```python
from build123d import *

# Parameters (mm, degrees)
SKETCH7_W           = 100
SKETCH7_H           = 14.5
BOSS_EXTRUDE1_DEPTH = 16.5
SKETCH8_R           = 4.75
CUT_EXTRUDE2_DEPTH  = 16
CUT_EXTRUDE3_START  = -2
SKETCH9_W           = 27
SKETCH9_H           = 27
CUT_EXTRUDE3_DEPTH  = 2
CUT_EXTRUDE4_DEPTH  = 2
FILLET1_R           = 3
FILLET2_R           = 3
FILLET3_R           = 0.3
FILLET4_R           = 3


with BuildPart() as part:
    # Sketch7 → Boss-Extrude1 (new body)
    with BuildSketch(Plane(origin=(0, 0, 0), x_dir=(0, 1, 0), z_dir=(0, 0, 1))):
        Rectangle(SKETCH7_W, SKETCH7_H)
    extrude(amount=BOSS_EXTRUDE1_DEPTH)

    # Sketch8 → Cut-Extrude2 (cut)
    with BuildSketch(Plane(origin=(0, 0, 16.5), x_dir=(0, -1, 0), z_dir=(0, 0, 1))):
        with Locations(Location((0, 0, 0), (0, 0, 90))):
            Circle(SKETCH8_R)
    extrude(amount=-CUT_EXTRUDE2_DEPTH, mode=Mode.SUBTRACT)

    # Sketch9 → Cut-Extrude3 (cut)
    with BuildSketch(Plane.XY.offset(16.5).offset(CUT_EXTRUDE3_START)):
        with Locations((0, -35)):
            Rectangle(SKETCH9_W, SKETCH9_H)
    cut_extrude3 = extrude(amount=-CUT_EXTRUDE3_DEPTH, mode=Mode.SUBTRACT)

    # Sketch10 → Cut-Extrude4 (cut)
    with BuildSketch(Plane.XY.offset(16.5)):
        with BuildLine():
            Line((0, -28), (-7.25, -28))
            Line((-7.25, -28), (-7.25, -42))
            Line((-7.25, -42), (0, -42))
            ThreePointArc((0, -42), (7, -35), (0, -28))
        make_face()
    cut_extrude4 = extrude(amount=-CUT_EXTRUDE4_DEPTH, mode=Mode.SUBTRACT)

    # Mirror1: Cut-Extrude3 across plane
    add(cut_extrude3.mirror(Plane.ZX), mode=Mode.SUBTRACT)

    # Mirror2: Cut-Extrude4 across plane
    add(cut_extrude4.mirror(Plane.ZX), mode=Mode.SUBTRACT)

    # Fillet1
    fillet1_edges = [part.edges().sort_by_distance(p)[0] for p in [
        (-7.25, 0, 0),
    ]]
    fillet(fillet1_edges, radius=FILLET1_R)

    # Fillet2
    fillet2_edges = [part.edges().sort_by_distance(p)[0] for p in [
        (7.25, 0, 0),
    ]]
    fillet(fillet2_edges, radius=FILLET2_R)

    # Fillet3
    fillet3_edges = [part.edges().sort_by_distance(p)[0] for p in [
        (-4.75, 0, 16.5),
    ]]
    fillet(fillet3_edges, radius=FILLET3_R)

    # Fillet4
    # the kernel refuses this fillet: 3 mm, written as the material it takes off along each edge
    with BuildSketch(Plane(origin=(-4.25, -50, 3), x_dir=(0, 0, -1), z_dir=(1, 0, 0))) as fillet4_piece_1:
        with BuildLine():
            CenterArc((3 - FILLET4_R, FILLET4_R), FILLET4_R, 270, 90)
            Line((3, FILLET4_R), (3, 0))
            Line((3, 0), (3 - FILLET4_R, 0))
        make_face()
    revolve(axis=Axis((-4.25, -50, 3), (0, 1, 0)), revolution_arc=90, mode=Mode.SUBTRACT)
    with BuildSketch(Plane(origin=(-7.25, -50, 3), x_dir=(0, 1, 0), z_dir=(0, 0, 1))) as fillet4_piece_2:
        with BuildLine():
            CenterArc((FILLET4_R, -FILLET4_R), FILLET4_R, 90, 90)
            Line((0, -FILLET4_R), (0, 0))
            Line((0, 0), (FILLET4_R, 0))
        make_face()
    extrude(amount=21, mode=Mode.SUBTRACT)
    with BuildSketch(Plane(origin=(-14.75, -50, 16.5), x_dir=(0, 1, 0), z_dir=(1, 0, 0)), Plane(origin=(14.75, 50, 16.5), x_dir=(0, -1, 0), z_dir=(-1, 0, 0))) as fillet4_piece_3:
        with BuildLine():
            CenterArc((FILLET4_R, -FILLET4_R), FILLET4_R, 90, 90)
            Line((0, -FILLET4_R), (0, 0))
            Line((0, 0), (FILLET4_R, 0))
        make_face()
    extrude(amount=29.5, mode=Mode.SUBTRACT)
    with BuildSketch(Plane(origin=(7.25, -50, 3), x_dir=(0, 1, 0), z_dir=(0, 0, 1)), Plane(origin=(-7.25, 50, 3), x_dir=(0, -1, 0), z_dir=(0, 0, 1)), Plane(origin=(7.25, 50, 3), x_dir=(-1, 0, 0), z_dir=(0, 0, 1))) as fillet4_piece_4:
        with BuildLine():
            CenterArc((FILLET4_R, FILLET4_R), FILLET4_R, 180, 90)
            Line((0, FILLET4_R), (0, 0))
            Line((0, 0), (FILLET4_R, 0))
        make_face()
    extrude(amount=21, mode=Mode.SUBTRACT)
    with BuildSketch(Plane(origin=(4.25, -50, 3), x_dir=(0, 0, -1), z_dir=(-1, 0, 0))) as fillet4_piece_5:
        with BuildLine():
            CenterArc((3 - FILLET4_R, -FILLET4_R), FILLET4_R, 0, 90)
            Line((3, -FILLET4_R), (3, 0))
            Line((3, 0), (3 - FILLET4_R, 0))
        make_face()
    revolve(axis=Axis((4.25, -50, 3), (0, -1, 0)), revolution_arc=90, mode=Mode.SUBTRACT)
    with BuildSketch(Plane(origin=(-4.25, -50, 0), x_dir=(0, 0, 1), z_dir=(1, 0, 0)), Plane(origin=(4.25, 50, 0), x_dir=(0, 0, 1), z_dir=(-1, 0, 0))) as fillet4_piece_6:
        with BuildLine():
            CenterArc((FILLET4_R, -FILLET4_R), FILLET4_R, 90, 90)
            Line((0, -FILLET4_R), (0, 0))
            Line((0, 0), (FILLET4_R, 0))
        make_face()
    extrude(amount=8.5, mode=Mode.SUBTRACT)
    with BuildSketch(Plane(origin=(-4.25, 50, 3), x_dir=(0, 0, -1), z_dir=(1, 0, 0))) as fillet4_piece_7:
        with BuildLine():
            CenterArc((3 - FILLET4_R, -FILLET4_R), FILLET4_R, 0, 90)
            Line((3, -FILLET4_R), (3, 0))
            Line((3, 0), (3 - FILLET4_R, 0))
        make_face()
    revolve(axis=Axis((-4.25, 50, 3), (0, 1, 0)), revolution_arc=90, mode=Mode.SUBTRACT)
    with BuildSketch(Plane(origin=(4.25, 50, 3), x_dir=(0, 0, -1), z_dir=(-1, 0, 0))) as fillet4_piece_8:
        with BuildLine():
            CenterArc((3 - FILLET4_R, FILLET4_R), FILLET4_R, 270, 90)
            Line((3, FILLET4_R), (3, 0))
            Line((3, 0), (3 - FILLET4_R, 0))
        make_face()
    revolve(axis=Axis((4.25, 50, 3), (0, -1, 0)), revolution_arc=90, mode=Mode.SUBTRACT)


solid = part.part
```
Geometry: final body of the model. Coordinates: model frame, mm. A direction names the side the tool comes from. Coordinates: 2 decimals unless noted, no trailing zeros. Order: outer loops, then holes, each group sorted by start corner. A loop starts at its lowest first (then second) coordinate and runs counter-clockwise, first axis right, second up. Notation, with made-up numbers: (73, 32) -> (113, 32) arc R25 cw to (113, 53) -> close; hole circle Ø7 at (23.25, 44.25). An arc over 180 degrees is marked (long way). Answer in a Markdown table with one row per item.
Item 1: Section C-C on y = 12. Output: boundary loops of the cut face in (x, z), plus the area to 3 significant figures.
Return value:
| item | result |
|---|---|
| outline | (-7.25, 3) arc R3 ccw to (-4.25, 0) -> (4.25, 0) arc R3 ccw to (7.25, 3) -> (7.25, 16.5) -> (-7.25, 16.5) -> close |
| area | 235 mm² |
Item 2: Section B-B on y = 35. Output: boundary loops of the cut face in (x, z), plus the area to 3 significant figures.
Return value:
| item | result |
|---|---|
| outline | (-7.25, 3) arc R3 ccw to (-4.25, 0) -> (4.25, 0) arc R3 ccw to (7.25, 3) -> (7.25, 12.5) -> (-7.25, 12.5) -> close; (7, 14.5) -> (7.25, 14.5) -> (7.25, 16.5) -> (7, 16.5) -> close |
| area | 178 mm² |
Item 3: Contact query for flat-ended pins moving along their axis: P1, Ø2, axis at x = -4, z = 16, coming from the +Y side; P2, Ø1, axis at x = -2.5, z = 15.5, coming from the -Y side; P3, Ø2, axis at x = -2.5, z = 15.5, coming from the -Y side. Output: stop coordinate, or through.
Return value:
| item | result |
|---|---|
| P1 | stops at y = 49.6 |
| P2 | stops at y = -49.6 |
| P3 | stops at y = -49.83 |
Item 4: Draft query along Z for faces 4 (the flat face through (0, 50, 8)), 5 (the flat face through (0, -1, 0)), 6 (the flat face through (0, -35, 12.5)). Return one class per face: released by +Z, released by -Z, zero draft, split by the parting line, or undercut.
Return value:
| item | result |
|---|---|
| face 4 | zero draft |
| face 5 | released by -Z |
| face 6 | undercut |
Item 5: Section A-A on z = 9.75. Output: boundary loops of the cut face in (x, y), plus the area to 3 significant figures.
Return value:
| item | result |
|---|---|
| outline | (-7.25, -47) arc R3 ccw to (-4.25, -50) -> (4.25, -50) arc R3 ccw to (7.25, -47) -> (7.25, 47) arc R3 ccw to (4.25, 50) -> (-4.25, 50) arc R3 ccw to (-7.25, 47) -> close; hole circle Ø9.5 at (0, 0) |
| area | 1,370 mm² |
Item 6: Ray query, L1, parallel to Y at x = 0, z = 12; L2, parallel to Z at x = 4.25, y = -28.5; L3, parallel to Y at x = 3.25, z = 13. Return the intervals inside material, ascending.
Return value:
| item | result |
|---|---|
| L1 | y = -50 to -4.75, 4.75 to 50 |
| L2 | z = 0 to 12.5, 14.5 to 16.5 |
| L3 | y = -50 to -48.5, -21.5 to -3.46, 3.46 to 21.5, 48.5 to 50 |
Item 7: Access query for faces 1 (the cylindrical face through (6.39, 49.1, 8.16)), 2 (the flat face through (0, -48.5, 14)), 3 (the cylindrical face through (7, 35, 16)). Directions: +Z, -Z, +X, -X, +Y, -Y. A direction counts if a zero-diameter tool reaches every point of the face in a straight line with its end or side. Return the directions, or none.
Return value:
| item | result |
|---|---|
| face 1 | +Z, -Z, +X, +Y |
| face 2 | +X, -X |
| face 3 | +Z, -X |
Item 8: Section D-D on y = -33.5. Output: boundary loops of the cut face in (x, z), plus the area to 3 significant figures.
Return value:
| item | result |
|---|---|
| outline | (-7.25, 3) arc R3 ccw to (-4.25, 0) -> (4.25, 0) arc R3 ccw to (7.25, 3) -> (7.25, 12.5) -> (-7.25, 12.5) -> close; (6.84, 14.5) -> (7.25, 14.5) -> (7.25, 16.5) -> (6.84, 16.5) -> close |
| area | 178 mm² |
